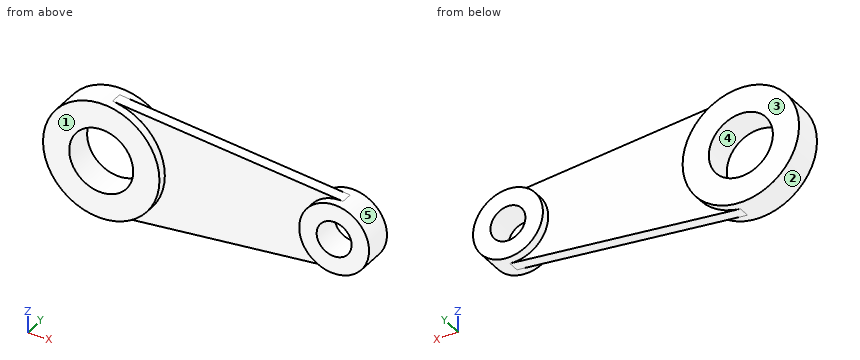
```python
from build123d import *

# Parameters (mm, degrees)
F1_DEPTH = 5
F0_R     = 27.5
F0_R_2   = 15
F2_DEPTH = 12.5


with BuildPart() as f1:
    # F0 (on Front) → F1 (new body, symmetric)
    with BuildSketch(Plane.XZ):
        with BuildLine():
            ThreePointArc((-195, 49.7493718553), (-162.9190075645, 33.5410196625), (-150, 0))
            ThreePointArc((-150, 0), (-162.9190075645, -33.5410196625), (-195, -49.7493718553))
            Line((-195, -49.7493718553), (3, -29.8496231132))
            ThreePointArc((3, -29.8496231132), (-30, 0), (3, 29.8496231132))
            Line((3, 29.8496231132), (-195, 49.7493718553))
        make_face()
    extrude(amount=F1_DEPTH, both=True)

    # F0 (on Front) → F2 (join, symmetric)
    with BuildSketch(Plane.XZ):
        with BuildLine():
            ThreePointArc((-195, -49.7493718553), (-162.9190075645, -33.5410196625), (-150, 0))
            ThreePointArc((-150, 0), (-162.9190075645, 33.5410196625), (-195, 49.7493718553))
            ThreePointArc((-195, 49.7493718553), (-250, 0), (-195, -49.7493718553))
        make_face()
        with Locations((-200, 0)):
            Circle(F0_R, mode=Mode.SUBTRACT)
        with BuildLine():
            ThreePointArc((30, 0), (22.2485954613, 20.1246117975), (3, 29.8496231132))
            ThreePointArc((3, 29.8496231132), (-30, 0), (3, -29.8496231132))
            ThreePointArc((3, -29.8496231132), (22.2485954613, -20.1246117975), (30, 0))
        make_face()
        Circle(F0_R_2, mode=Mode.SUBTRACT)
    extrude(amount=F2_DEPTH, both=True)


solid = f1.part
```
Verification items for the finished model (mm, model axes). Face numbers are marked on the shaded views. A direction names the side the tool comes from. Round coordinates to 2 decimals unless told otherwise and drop trailing zeros. Order: outer loops, then holes, each group sorted by start corner. A loop starts at its lowest first (then second) coordinate and runs counter-clockwise, first axis right, second up. Notation, with made-up numbers: (-26.75, 6) - (10.25, 6) arc R15 cw to (10.25, 10) - close; hole circle Ø5 at (29.25, 74). An arc over 180 degrees is marked (long way). Use CSV: the item, a comma, the result in double quotes. Start each with the question number.
1) Go/stop test with flat-tipped pins: P1, Ø2, axis at x = -216, y = 6.5, coming from the -Z side; P2, Ø1, axis at x = -24.5, y = 10, coming from the -Z side; P3, Ø4, axis at y = -2.5, z = -15, coming from the +X side. Record where each tip stops, or that it passes through.
2) Section check A-A, the plane z = 0. Record the cut outline in (x, y), plus the area to 4 significant figures.
3) Mould release check, pull along Z, two halves, no side actions. Record for the marked faces 3, 4 and 5: +Z half, -Z half, draft (parallel to the pull), parting line (faces both ways), or undercut.
4) Section check C-C, the plane y = 0.25. Record the cut outline in (x, z), plus the area to 3 significant figures.
5) Access from +Z, -Z, +X, -X, +Y, -Y to the whole of each face (thin tool, end or side, straight path). Record for the marked faces 1 and 2.
6) Section check D-D, the plane z = 25. Record the cut outline in (x, y).
7) Thickness scan on L1, parallel to X at y = 11, z = -3; L2, parallel to Z at x = -200, y = -5.25; L3, parallel to Y at x = -39.5, z = -27. Record the ranges inside material, lowest first.
8) Section check B-B, the plane x = -200. Record the cut outline in (y, z), plus the area to 4 significant figures.
Answers:
1,P1,"stops at z = -47.7"
1,P2,"stops at z = -18"
1,P3,"stops at x = 27.04"
2,outline,"(-250, -12.5) - (-227.5, -12.5) - (-227.5, 12.5) - (-250, 12.5) - close; (-172.5, -12.5) - (-150, -12.5) - (-150, -5) - (-30, -5) - (-30, -12.5) - (-15, -12.5) - (-15, 12.5) - (-30, 12.5) - (-30, 5) - (-150, 5) - (-150, 12.5) - (-172.5, 12.5) - close; (15, -12.5) - (30, -12.5) - (30, 12.5) - (15, 12.5) - close"
2,area,"3,075 mm²"
3,face 3,"draft"
3,face 4,"undercut"
3,face 5,"parting line"
4,outline,"(-195, -49.75) - (3, -29.85) arc R30 ccw to (3, 29.85) - (-195, 49.75) arc R50 ccw (long way) to start; hole circle Ø55 at (-200, 0); hole circle Ø30 at (0, 0)"
4,area,"18,300 mm²"
5,face 1,"+Z, -Z, +X, -X, -Y"
5,face 2,"none"
6,outline,"(-243.3, -12.5) - (-211.46, -12.5) - (-211.46, 12.5) - (-243.3, 12.5) - close; (-188.54, -12.5) - (-156.7, -12.5) - (-156.7, -5) - (-16.58, -5) - (-16.58, -12.5) - (16.58, -12.5) - (16.58, 12.5) - (-16.58, 12.5) - (-16.58, 5) - (-156.7, 5) - (-156.7, 12.5) - (-188.54, 12.5) - close"
7,L1,"x = -249.91 to -227.34, -172.66 to -150.09, -29.85 to -14.7, 14.7 to 29.85"
7,L2,"z = -50 to -27.5, 27.5 to 50"
7,L3,"y = -5 to 5"
8,outline,"(-12.5, -50) - (12.5, -50) - (12.5, -27.5) - (-12.5, -27.5) - close; (-12.5, 27.5) - (12.5, 27.5) - (12.5, 50) - (-12.5, 50) - close"
8,area,"1,125 mm²"
